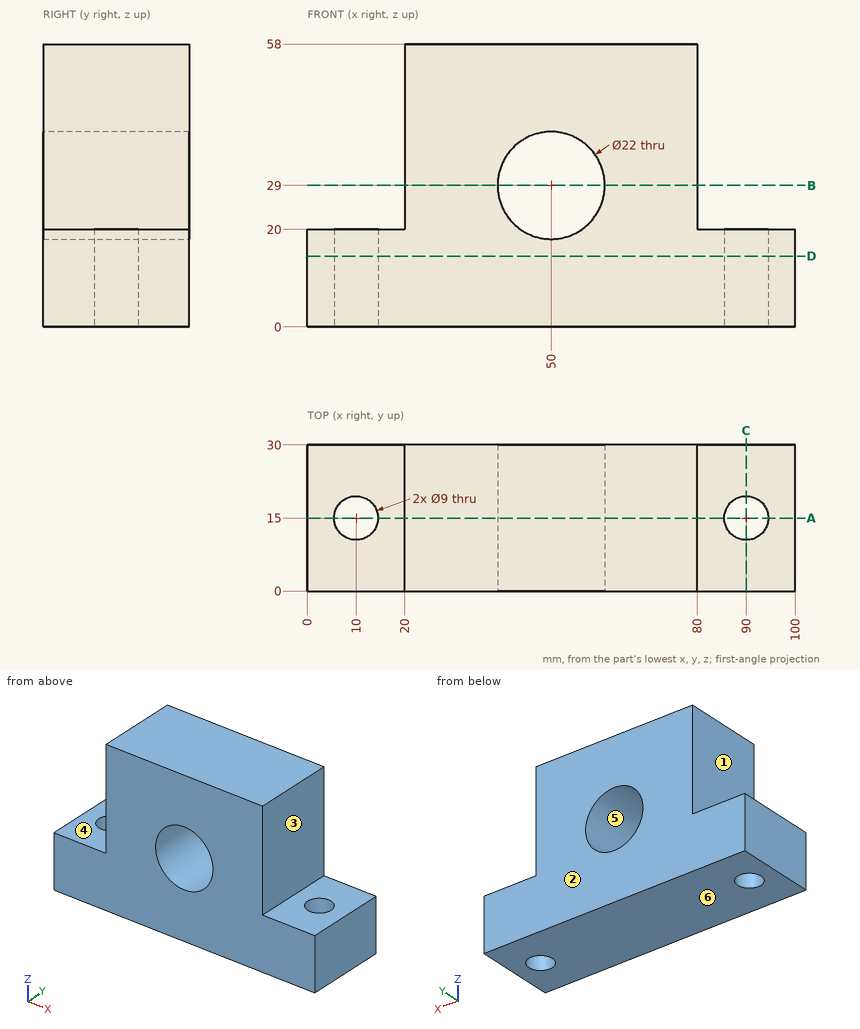
The figure shows three views and two pictorial views of one solid part (mm, origin at its lowest corner). Answer the questions. A direction names the side the tool comes from. Coordinates: 2 decimals unless noted, no trailing zeros. Loops run counter-clockwise (first coordinate to the right, second up) from the corner with the lowest first, then second, coordinate; pieces in that order, holes last.
1) Find section B-B on z = 29. Write down the section's boundary in (x, y), then the cut area to 3 significant figures.
2) Find the intervals of material crossed by L1, parallel to Y at x = 90, z = 14.5; L2, parallel to Z at x = 49.5, y = 22; L3, parallel to X at y = 11, z = 29, in increasing order.
3) Find section C-C on x = 90. Write down the section's boundary in (y, z), then the cut area to 3 significant figures.
4) A tool of negligible diameter and unlimited length cuts with its end or side. For the marked faces 1, 2 and 3, from which of +Z, -Z, +X, -X, +Y, -Y can it reach the whole face along a straight path? Write none if from no direction.
5) Flat-ended cylindrical pins translate along their axes: pin 1 Ø10.5 at (x, y) = (10, 15) entering from +Z; pin 2 Ø8 at (x, y) = (90, 15) entering from +Z; pin 3 Ø5 at (y, z) = (17.5, 46) entering from -X. Find the tip coordinate at first contact, or state that the pin passes through.
6) Find section A-A on y = 15. Write down the section's boundary in (x, z), then the cut area to 3 significant figures.
7) Find section D-D on z = 14.5. Write down the section's boundary in (x, y), then the cut area to 3 significant figures.
8) Determine the mould class of the marked faces 4, 5 and 6 for opening direction Z: pulls with the +Z half, pulls with the -Z half, needs draft (parallel to the pull), parting line crosses it, or undercut.
Values:
1. outline: (20, 0) - (39, 0) - (39, 30) - (20, 30) - close; (61, 0) - (80, 0) - (80, 30) - (61, 30) - close
1. area: 1,140 mm2
2. L1: y = 0 to 10.5, 19.5 to 30
2. L2: z = 0 to 18.01, 39.99 to 58
2. L3: x = 20 to 39, 61 to 80
3. outline: (0, 0) - (10.5, 0) - (10.5, 20) - (0, 20) - close; (19.5, 0) - (30, 0) - (30, 20) - (19.5, 20) - close
3. area: 420 mm2
4. face 1: +Z, -X, +Y, -Y
4. face 2: +Z, -Z, +X, -X, +Y
4. face 3: +Z, +X, +Y, -Y
5. pin 1: stops at z = 20
5. pin 2: passes through
5. pin 3: stops at x = 20
6. outline: (0, 0) - (5.5, 0) - (5.5, 20) - (0, 20) - close; (14.5, 0) - (85.5, 0) - (85.5, 20) - (80, 20) - (80, 58) - (20, 58) - (20, 20) - (14.5, 20) - close; (94.5, 0) - (100, 0) - (100, 20) - (94.5, 20) - close; hole circle Ø22 at (50, 29)
6. area: 3,540 mm2
7. outline: (0, 0) - (100, 0) - (100, 30) - (0, 30) - close; hole circle Ø9 at (10, 15); hole circle Ø9 at (90, 15)
7. area: 2,870 mm2
8. face 4: pulls with the +Z half
8. face 5: undercut
8. face 6: pulls with the -Z half
